For this review, take the finished solid that the model builds, in its own axes (mm). Coordinates: 2 decimals unless noted, no trailing zeros. Loops run counter-clockwise (first coordinate to the right, second up) from the corner with the lowest first, then second, coordinate; pieces in that order, holes last. Notation, with made-up numbers: M -3,87.5 L 49,87.5 A15 cw 49,109.5 Z; hole C -24.75,65.25 d6. An arc over 180 degrees is marked long. Use one line per item in the form item = value.
```python
from build123d import *

# Parameters (mm, degrees)
SKETCH1_W           = 42.3
SKETCH1_H           = 42.3
BOSS_EXTRUDE2_DEPTH = 5
SKETCH2_R           = 3
CUT_EXTRUDE1_DEPTH  = 5
CIRPATTERN1_COUNT   = 4


with BuildPart() as part:
    # Sketch1 → Boss-Extrude2 (new body)
    with BuildSketch(Plane(origin=(0, 0, 0), x_dir=(1, 0, 0), z_dir=(0, 1, 0))):
        Rectangle(SKETCH1_W, SKETCH1_H)
    extrude(amount=BOSS_EXTRUDE2_DEPTH)

    # Sketch2 → Cut-Extrude1 (cut)
    with BuildSketch(Plane(origin=(0, 5, 0), x_dir=(1, 0, 0), z_dir=(0, 1, 0))):
        with Locations(Location((-17.127358159, 17.127358159, 0), (0, 0, 270))):
            Circle(SKETCH2_R)
    cut_extrude1 = extrude(amount=-CUT_EXTRUDE1_DEPTH, mode=Mode.SUBTRACT)

    # CirPattern1: Cut-Extrude1 ×4 about axis
    cirpattern1_axis = Axis((0.274991672, 0, 0.274991672), (0, 1, 0))
    for i in range(1, CIRPATTERN1_COUNT):
        add(cut_extrude1.rotate(cirpattern1_axis, i * 360 / CIRPATTERN1_COUNT), mode=Mode.SUBTRACT)


solid = part.part
```
1. Wall thickness on line 1 along X through (y, z) = (1.45, 15); line 2 along Z through (x, y) = (18, 2.5); line 3 along X through (y, z) = (1.35, 16.5): over which ranges is each line inside the solid? List them lowest first. Write a range as from..to.
Computed values:
line_1 = -21.15..-18.48, -15.77..16.32, 19.03..21.15
line_2 = -21.15..-20.11, -14.14..14.69, 20.66..21.15
line_3 = -21.15..-19.89, -14.37..14.92, 20.44..21.15
2. Consider section A-A on x = -16. Write out the cut boundary in (y, z), plus the area to 3 significant figures.
Computed values:
outline = M 0,-21.15 L 5,-21.15 L 5,-19.91 L 0,-19.91 Z; M 0,-14.35 L 5,-14.35 L 5,14.9 L 0,14.9 Z; M 0,20.46 L 5,20.46 L 5,21.15 L 0,21.15 Z
area = 156 mm2
3. Consider section B-B on z = 19. Write out the cut boundary in (x, y).
Computed values:
outline = M -21.15,0 L -19.82,0 L -19.82,5 L -21.15,5 Z; M -14.43,0 L 14.98,0 L 14.98,5 L -14.43,5 Z; M 20.37,0 L 21.15,0 L 21.15,5 L 20.37,5 Z
4. Consider section C-C on y = 1.65. Write out the cut boundary in (x, z), plus the area to 3 significant figures.
Computed values:
outline = M -21.15,-21.15 L 21.15,-21.15 L 21.15,21.15 L -21.15,21.15 Z; hole C -17.13,-17.13 d6; hole C -17.13,17.68 d6; hole C 17.68,-17.13 d6; hole C 17.68,17.68 d6
area = 1,680 mm2
5. Draft analysis for pull direction Z (two halves, no side actions). For faces 1 (the face through (-18.276, 2.535, -14.356)), 2 (the face through (21.15, 2, 0)), 3 (the face through (0, 2, 21.15)), state which applies: +Z half, -Z half, draft (parallel to the pull), parting line (faces both ways), or undercut.
Computed values:
face_1 = undercut
face_2 = draft
face_3 = +Z half
